Work out the finished part from the listing and answer in its coordinate system (mm). A direction names the side the tool comes from. Round coordinates to 2 decimals unless told otherwise and drop trailing zeros. Order: outer loops, then holes, each group sorted by start corner. A loop starts at its lowest first (then second) coordinate and runs counter-clockwise, first axis right, second up. Notation, with made-up numbers: (-11, 24.25) - (5, 24.25) arc R35 ccw to (5, 58.25) - close; hole circle Ø11 at (54, -37.75). An arc over 180 degrees is marked (long way). Answer in a Markdown table with one row per item.
from build123d import *

# Parameters (mm, degrees)
F3_DEPTH      = 6.35
F3_DEPTH_BACK = 1.271
F4_W          = 1.27
F4_H          = 76.2
F5_DEPTH      = 76.201
F5_DEPTH_BACK = 1.2710001


with BuildPart() as f1:
    # F0 (on Top) → F1 (revolve)
    with BuildSketch(Plane.XY):
        with BuildLine():
            Line((304.8, 5.08), (304.8, 76.2))
            Line((304.8, 76.2), (303.53, 76.2))
            Line((303.53, 76.2), (303.53, 5.08))
            ThreePointArc((303.53, 5.08), (305.3898719395, 0.5898719395), (309.88, -1.27))
            Line((309.88, -1.27), (330.2, -1.27))
            Line((330.2, -1.27), (330.2, 0))
            Line((330.2, 0), (309.88, 0))
            ThreePointArc((309.88, 0), (306.2878975516, 1.4878975516), (304.8, 5.08))
        make_face()
    revolve(axis=Axis((0, 33.4558707156, 0), (0, -1, 0)))

    # F2 (on Front) → F3 (cut, two sides)
    with BuildSketch(Plane.XZ) as f3_sk:
        with BuildLine():
            Line((162.6306192468, -256.2844954019), (175.976362049, -279.4))
            ThreePointArc((175.976362049, -279.4), (285.9615883296, -165.1), (329.9556788419, -12.7))
            Line((329.9556788419, -12.7), (303.2641932375, -12.7))
            ThreePointArc((303.2641932375, -12.7), (262.8646908107, -151.765), (162.6306192468, -256.2844954019))
        make_face()
        with BuildLine():
            Line((303.2641932375, 12.7), (329.9556788419, 12.7))
            ThreePointArc((329.9556788419, 12.7), (285.9615883296, 165.1), (175.976362049, 279.4))
            Line((175.976362049, 279.4), (162.6306192468, 256.2844954019))
            ThreePointArc((162.6306192468, 256.2844954019), (262.8646908107, 151.765), (303.2641932375, 12.7))
        make_face()
        with BuildLine():
            ThreePointArc((-140.6335739907, 268.9844954019), (0, 303.53), (140.6335739907, 268.9844954019))
            Line((140.6335739907, 268.9844954019), (153.9793167929, 292.1))
            ThreePointArc((153.9793167929, 292.1), (0, 330.2), (-153.9793167929, 292.1))
            Line((-153.9793167929, 292.1), (-140.6335739907, 268.9844954019))
        make_face()
        with BuildLine():
            Line((-329.9556788419, 12.7), (-303.2641932375, 12.7))
            ThreePointArc((-303.2641932375, 12.7), (-262.8646908107, 151.765), (-162.6306192468, 256.2844954019))
            Line((-162.6306192468, 256.2844954019), (-175.976362049, 279.4))
            ThreePointArc((-175.976362049, 279.4), (-285.9615883296, 165.1), (-329.9556788419, 12.7))
        make_face()
        with BuildLine():
            Line((-175.976362049, -279.4), (-162.6306192468, -256.2844954019))
            ThreePointArc((-162.6306192468, -256.2844954019), (-262.8646908107, -151.765), (-303.2641932375, -12.7))
            Line((-303.2641932375, -12.7), (-329.9556788419, -12.7))
            ThreePointArc((-329.9556788419, -12.7), (-285.9615883296, -165.1), (-175.976362049, -279.4))
        make_face()
        with BuildLine():
            ThreePointArc((-153.9793167929, -292.1), (0, -330.2), (153.9793167929, -292.1))
            Line((153.9793167929, -292.1), (140.6335739907, -268.9844954019))
            ThreePointArc((140.6335739907, -268.9844954019), (0, -303.53), (-140.6335739907, -268.9844954019))
            Line((-140.6335739907, -268.9844954019), (-153.9793167929, -292.1))
        make_face()
    extrude(amount=-F3_DEPTH, mode=Mode.SUBTRACT)
    extrude(f3_sk.sketch, amount=F3_DEPTH_BACK, mode=Mode.SUBTRACT)

    # F4 (on Front) → F5 (cut, two sides)
    with BuildSketch(Plane.XZ) as f5_sk:
        with Locations((0, -319.9747502804)):
            Rectangle(F4_W, F4_H)
    extrude(amount=-F5_DEPTH, mode=Mode.SUBTRACT)
    extrude(f5_sk.sketch, amount=F5_DEPTH_BACK, mode=Mode.SUBTRACT)


solid = f1.part
1) Find section C-C, the plane y = 61.5. Give the vertices of the cut face in (x, z) (3 decimals).
Filled in:
| item | result |
|---|---|
| outline | (-0.635, -304.799) - (-0.635, -303.529) arc R303.53 cw (long way) to (0.635, -303.529) - (0.635, -304.799) arc R304.8 ccw (long way) to start |
2) Find section B-B, the plane x = -220. Give the vertices of the cut face in (y, z).
Filled in:
| item | result |
|---|---|
| outline | (6.35, -210.96) - (76.2, -210.96) - (76.2, -209.12) - (6.35, -209.12) - close; (6.35, 209.12) - (76.2, 209.12) - (76.2, 210.96) - (6.35, 210.96) - close |
3) Which of the six approach directions +Z, -Z, +X, -X, +Y, -Y give full straight-line access (tool end or side, diameter ignored) to faces 1 (the face through (-160, 0, -277)), 2 (the face through (160, 0, 277)), 3 (the face through (320, 0, 0)), 4 (the face through (-320, 0, 0)), 5 (the face through (160, 0, -277))?
Filled in:
| item | result |
|---|---|
| face 1 | -Z, -X, +Y |
| face 2 | +Z, +X, +Y |
| face 3 | +Z, -Z, +X, +Y |
| face 4 | +Z, -Z, -X, +Y |
| face 5 | -Z, +X, +Y |
4) Find the intervals of material crossed by probe 1 along X at (y, z) = (32, 0); probe 2 along Z at (x, y) = (0, 25); probe 3 along Z at (x, y) = (-139, 25), in increasing order. Write a range as from..to.
Filled in:
| item | result |
|---|---|
| probe 1 | x = -304.8..-303.53, 303.53..304.8 |
| probe 2 | z = 303.53..304.8 |
| probe 3 | z = -271.26..-269.83, 269.83..271.26 |
5) Find section A-A, the plane z = -34. Give the vertices of the cut face in (x, y), then the cut area to 3 significant figures.
Filled in:
| item | result |
|---|---|
| outline | (-302.9, 6.35) - (-301.62, 6.35) - (-301.62, 76.2) - (-302.9, 76.2) - close; (301.62, 6.35) - (302.9, 6.35) - (302.9, 76.2) - (301.62, 76.2) - close |
| area | 179 mm^2 |
6) Each of these flat-tipped pins is pushed along its axis until it touches: pin 1 (22.5 mm diameter, centred on x = -323.5, z = 3, fed in from +Y); pin 2 (6 mm diameter, centred on x = 161.5, y = 42, fed in from -Z); pin 3 (1.5 mm diameter, centred on y = 7, z = 172.5, fed in from +X). Where does it stop, or does it pass through?
Filled in:
| item | result |
|---|---|
| pin 1 | stops at y = 0 |
| pin 2 | stops at z = -260.35 |
| pin 3 | stops at x = 251.8 |
